The listing builds one solid part. Answer for the finished solid, in the listing's coordinates (mm). A direction names the side the tool comes from. Round coordinates to 2 decimals unless told otherwise and drop trailing zeros. Order: outer loops, then holes, each group sorted by start corner. A loop starts at its lowest first (then second) coordinate and runs counter-clockwise, first axis right, second up. Notation, with made-up numbers: M -11.75,14.5 L 11.25,14.5 A22 ccw 11.25,24.5 Z; hole C 20,34 d10. An arc over 180 degrees is marked long. Put each result on its own line as item: value. Start each with the question number.
1. Each of these flat-tipped pins is pushed along its axis until it touches: pin 1 Ø25 at (x, y) = (-32, 25) entering from +Z; pin 2 Ø4 at (y, z) = (64, -99) entering from +X; pin 3 Ø1.8 at (y, z) = (62.5, 94.5) entering from +X; pin 4 Ø4 at (y, z) = (16.5, -66.5) entering from +X. Where does it stop, or does it pass through?
2. The part is cut by section B-B (y = 43). Give the vertices of the cut face in (x, z).
3. The part is cut by section A-A (x = -22). Give the vertices of the cut face in (y, z).
4. The mould has two halves that part along Z. Classify faces 4 (the face through (-4.9, 64.4, -115)), 5 (the face through (-25, 63.6, 97)), 6 (the face through (69.983, 33.18, 1.539)), 7 (the face through (10, 1.6, -1)): +Z half, -Z half, draft (parallel to the pull), parting line (faces both ways), or undercut.
5. Which of the six approach directions +Z, -Z, +X, -X, +Y, -Y give full straight-line access (tool end or side, diameter ignored) to faces 1 (the face through (-25, 33, -70)), 2 (the face through (-25, 32, -71.6)), 3 (the face through (-25, 33, 71.6))?
6. Consider line 1 (Z direction, x = -19, y = 60); line 2 (Y direction, x = 64, z = 24); line 3 (Z direction, x = 51, y = 24.5). Determine where each line is inside the solid, lowest interval first.
from build123d import *

# Parameters (mm, degrees)
SM_BASE_FLANGE_2_DEPTH             = 1.6
SM_START                           = -50
SM_EDGE_FLANGE_2_DEPTH             = 121.6
SM_EDGE_FLANGE_2_2_DEPTH           = 50
SM_EDGE_FLANGE_2_3_ANGLE           = 180
SM_EDGE_FLANGE_2_4_ANGLE           = 180
SM_EDGE_FLANGE_3_STRIP_W           = 10.4
SM_EDGE_FLANGE_3_STRIP_H           = 1.6
SM_EDGE_FLANGE_3_STRIP_CUT_DEPTH   = 50
SM_EDGE_FLANGE_3_STRIP_2_W         = 10.4
SM_EDGE_FLANGE_3_STRIP_2_H         = 1.6
SM_EDGE_FLANGE_3_STRIP_CUT_2_DEPTH = 50
SM_EDGE_FLANGE_3_DEPTH             = 50
SM_EDGE_FLANGE_3_BEND_DEPTH        = 50
CHAMFER_1_SIZE                     = 10
CUT_EXTRUDE_1_REACH                = 155.608


with BuildPart() as part:
    # 基材-凸緣2: sheet metal written as solids
    # 草圖6 → 基材-凸緣2 (new body)
    with BuildSketch(Plane(origin=(0, 0, 0), x_dir=(1, 0, 0), z_dir=(0, 1, 0))):
        with BuildLine():
            Line((-50, 70), (0, 70))
            ThreePointArc((0, 70), (70, 0), (0, -70))
            Line((0, -70), (-50, -70))
            Line((-50, -70), (-50, 70))
        make_face()
    extrude(amount=SM_BASE_FLANGE_2_DEPTH)

    # 邊線-凸緣2: read off the stored shape, not the designer's step
    # 邊線-凸緣2 outline → 邊線-凸緣2 (cut)
    with BuildSketch(Plane.YZ.offset(SM_START)):
        with BuildLine():
            ThreePointArc((0, 68), (0.155005568, 69.044994432), (0.606674091, 70))
            Line((0.606674091, 70), (0, 70))
            Line((0, 70), (0, 68))
        make_face()
        with BuildLine():
            Line((0, -70), (0.606674091, -70))
            ThreePointArc((0.606674091, -70), (0.155005568, -69.044994432), (0, -68))
            Line((0, -68), (0, -70))
        make_face()
    extrude(amount=SM_EDGE_FLANGE_2_DEPTH, mode=Mode.SUBTRACT)

    # Sm Edge Flange 2 2 outline → Sm Edge Flange 2 2 (add)
    with BuildSketch(Plane.YZ.offset(SM_START)):
        with BuildLine():
            Line((3.6, 70), (63.6, 70))
            Line((63.6, 70), (63.6, 71.6))
            Line((63.6, 71.6), (3.6, 71.6))
            ThreePointArc((3.6, 71.6), (1.902943725, 71.174901573), (0.606674091, 70))
            Line((0.606674091, 70), (1.6, 70))
            Line((1.6, 70), (1.6, 68))
            ThreePointArc((1.6, 68), (2.185786438, 69.414213562), (3.6, 70))
        make_face()
        with BuildLine():
            Line((63.6, -71.6), (63.6, -70))
            Line((63.6, -70), (3.6, -70))
            ThreePointArc((3.6, -70), (2.185786438, -69.414213562), (1.6, -68))
            Line((1.6, -68), (1.6, -70))
            Line((1.6, -70), (0.606674091, -70))
            ThreePointArc((0.606674091, -70), (1.902943725, -71.174901573), (3.6, -71.6))
            Line((3.6, -71.6), (63.6, -71.6))
        make_face()
    extrude(amount=SM_EDGE_FLANGE_2_2_DEPTH)

    # Sm Edge Flange 2 3 outline → Sm Edge Flange 2 3 (revolve, cut)
    with BuildSketch(Plane.ZY):
        with BuildLine():
            ThreePointArc((70, 0.606674091), (69.044994432, 0.155005568), (68, 0))
            Line((68, 0), (70, 0))
            Line((70, 0), (70, 0.606674091))
        make_face()
    revolve(axis=Axis((0, 0, 0), (0, 1, 0)), revolution_arc=SM_EDGE_FLANGE_2_3_ANGLE, mode=Mode.SUBTRACT)

    # Sm Edge Flange 2 4 outline → Sm Edge Flange 2 4 (revolve)
    with BuildSketch(Plane.ZY):
        with BuildLine():
            Line((71.6, 63.6), (70, 63.6))
            Line((70, 63.6), (70, 3.6))
            ThreePointArc((70, 3.6), (69.414213562, 2.185786438), (68, 1.6))
            Line((68, 1.6), (70, 1.6))
            Line((70, 1.6), (70, 0.606674091))
            ThreePointArc((70, 0.606674091), (71.174901573, 1.902943725), (71.6, 3.6))
            Line((71.6, 3.6), (71.6, 63.6))
        make_face()
    revolve(axis=Axis((0, 0, 0), (0, 1, 0)), revolution_arc=SM_EDGE_FLANGE_2_4_ANGLE)

    # 邊線-凸緣3: sheet metal written as solids
    # 邊線-凸緣3 strip (on a plane across the edge) → 邊線-凸緣3 strip cut (cut)
    with BuildSketch(Plane(origin=(0, 63.6, 71.6), x_dir=(0, -1, 0), z_dir=(-1, 0, 0))):
        with Locations((-3.2, -0.8)):
            Rectangle(SM_EDGE_FLANGE_3_STRIP_W, SM_EDGE_FLANGE_3_STRIP_H)
    extrude(amount=SM_EDGE_FLANGE_3_STRIP_CUT_DEPTH, mode=Mode.SUBTRACT)

    # 邊線-凸緣3 strip 2 (on a plane across the edge) → 邊線-凸緣3 strip cut 2 (cut)
    with BuildSketch(Plane(origin=(-50, 63.6, -71.6), x_dir=(0, -1, 0), z_dir=(1, 0, 0))):
        with Locations((-3.2, -0.8)):
            Rectangle(SM_EDGE_FLANGE_3_STRIP_2_W, SM_EDGE_FLANGE_3_STRIP_2_H)
    extrude(amount=SM_EDGE_FLANGE_3_STRIP_CUT_2_DEPTH, mode=Mode.SUBTRACT)

    # 邊線-凸緣3 section (on a plane across the edge) → 邊線-凸緣3 (add)
    with BuildSketch(Plane(origin=(0, 63.6, 71.6), x_dir=(0, -1, 0), z_dir=(-1, 0, 0))):
        with BuildLine():
            Line((-1.6, 2), (-1.6, 48.5))
            Line((-1.6, 48.5), (0, 48.5))
            Line((0, 48.5), (0, 2))
            ThreePointArc((0, 2), (0.585786438, 0.585786438), (2, 0))
            Line((2, 0), (2, -1.6))
            ThreePointArc((2, -1.6), (-0.545584412, -0.545584412), (-1.6, 2))
        make_face()
    extrude(amount=SM_EDGE_FLANGE_3_DEPTH)

    # 邊線-凸緣3 section 2 (on a plane across the edge) → 邊線-凸緣3 bend (add)
    with BuildSketch(Plane(origin=(-50, 63.6, -71.6), x_dir=(0, -1, 0), z_dir=(1, 0, 0))):
        with BuildLine():
            Line((-1.6, 2), (-1.6, 48.5))
            Line((-1.6, 48.5), (0, 48.5))
            Line((0, 48.5), (0, 2))
            ThreePointArc((0, 2), (0.585786438, 0.585786438), (2, 0))
            Line((2, 0), (2, -1.6))
            ThreePointArc((2, -1.6), (-0.545584412, -0.545584412), (-1.6, 2))
        make_face()
    extrude(amount=SM_EDGE_FLANGE_3_BEND_DEPTH)

    # 導角1
    chamfer_1_edges = [part.edges().sort_by_distance(p)[0] for p in [
        (0, 64.4, 120.1),
        (-50, 64.4, 120.1),
        (-50, 64.4, -120.1),
        (0, 64.4, -120.1),
    ]]
    chamfer(chamfer_1_edges, length=CHAMFER_1_SIZE)

    # 草圖18 → 除料-伸長1 (cut, up to next)
    with BuildSketch(Plane.XZ.offset(-63.6), mode=Mode.PRIVATE) as cut_extrude_1_sk1:
        with BuildLine():
            Line((-35, 97.4), (-15, 97.4))
            ThreePointArc((-15, 97.4), (-12.3, 100.1), (-15, 102.8))
            Line((-15, 102.8), (-35, 102.8))
            ThreePointArc((-35, 102.8), (-37.7, 100.1), (-35, 97.4))
        make_face()
    cut_extrude_1_tool1 = extrude(cut_extrude_1_sk1.sketch, amount=-CUT_EXTRUDE_1_REACH, mode=Mode.PRIVATE) & part.part
    # 草圖18 → 除料-伸長1 (cut, up to next)
    with BuildSketch(Plane.XZ.offset(-63.6), mode=Mode.PRIVATE) as cut_extrude_1_sk2:
        with BuildLine():
            Line((-35, -102.8), (-15, -102.8))
            ThreePointArc((-15, -102.8), (-12.3, -100.1), (-15, -97.4))
            Line((-15, -97.4), (-35, -97.4))
            ThreePointArc((-35, -97.4), (-37.7, -100.1), (-35, -102.8))
        make_face()
    cut_extrude_1_tool2 = extrude(cut_extrude_1_sk2.sketch, amount=-CUT_EXTRUDE_1_REACH, mode=Mode.PRIVATE) & part.part
    add(cut_extrude_1_tool1.solids().sort_by_distance((-25, 63.6, 100.1))[0], mode=Mode.SUBTRACT)
    add(cut_extrude_1_tool2.solids().sort_by_distance((-25, 63.6, -100.1))[0], mode=Mode.SUBTRACT)


solid = part.part
Resolved:
1. pin 1: z = 71.6
1. pin 2: x = 0
1. pin 3: through
1. pin 4: x = 31.09
2. outline: M -50,-71.6 L 0,-71.6 A71.6 ccw 0,71.6 L -50,71.6 L -50,70 L 0,70 A70 cw 0,-70 L -50,-70 Z
3. outline: M 0,-68 A3.6 ccw 3.6,-71.6 L 61.6,-71.6 A2 cw 63.6,-73.6 L 63.6,-97.4 L 65.2,-97.4 L 65.2,-73.6 A3.6 ccw 61.6,-70 L 3.6,-70 A2 cw 1.6,-68 L 1.6,68 A2 cw 3.6,70 L 61.6,70 A3.6 ccw 65.2,73.6 L 65.2,97.4 L 63.6,97.4 L 63.6,73.6 A2 cw 61.6,71.6 L 3.6,71.6 A3.6 ccw 0,68 Z; M 63.6,-120.1 L 65.2,-120.1 L 65.2,-102.8 L 63.6,-102.8 Z; M 63.6,102.8 L 65.2,102.8 L 65.2,120.1 L 63.6,120.1 Z
4. face 4: -Z half
4. face 5: draft
4. face 6: undercut
4. face 7: undercut
5. face 1: -X, +Y
5. face 2: -Z, +X, -X, -Y
5. face 3: +Z, +X, -X, -Y
6. line 1: -71.6 to -70, 70 to 71.6
6. line 2: 0.02 to 1.63
6. line 3: -50.25 to -47.95, 47.95 to 50.25
